from build123d import *

# Parameters (mm, degrees)
SKETCH1_R           = 12.5
BOSS_EXTRUDE1_DEPTH = 150
BOSS_EXTRUDE2_START = 5
SKETCH3_R           = 15.5
BOSS_EXTRUDE2_DEPTH = 10
CIRPATTERN1_COUNT   = 7
FILLET1_R           = 1


with BuildPart() as part:
    # Sketch1 → Boss-Extrude1 (new body)
    with BuildSketch(Plane(origin=(0, 0, 0), x_dir=(1, 0, 0), z_dir=(0, 1, 0))):
        Circle(SKETCH1_R)
    extrude(amount=BOSS_EXTRUDE1_DEPTH)

    # Sketch3 → Boss-Extrude2 (add)
    with BuildSketch(Plane(origin=(0, 0, 0), x_dir=(1, 0, 0), z_dir=(0, 1, 0)).offset(BOSS_EXTRUDE2_START)):
        with BuildLine():
            Line((-2.253835774, 56.947383215), (-2.253835774, 12.295130105))
            Line((-2.253835774, 12.295130105), (2.253835774, 12.295130105))
            Line((2.253835774, 12.295130105), (2.253835774, 56.947383215))
            ThreePointArc((2.253835774, 56.947383215), (0, 92.805720885), (-2.253835774, 56.947383215))
        make_face()
        with Locations((0, 74.805720885)):
            Circle(SKETCH3_R, mode=Mode.SUBTRACT)
    boss_extrude2 = extrude(amount=BOSS_EXTRUDE2_DEPTH)

    # CirPattern1: Boss-Extrude2 ×7 about axis
    cirpattern1_axis = Axis((0, 0, 0), (0, 1, 0))
    for i in range(1, CIRPATTERN1_COUNT):
        add(boss_extrude2.rotate(cirpattern1_axis, i * 360 / CIRPATTERN1_COUNT))

    # Fillet1
    fillet1_edges = [part.edges().sort_by_distance(p)[0] for p in [
        (-12.5, 0, 0),
    ]]
    fillet(fillet1_edges, radius=FILLET1_R)


solid = part.part
Can you work these out from the model? Positions are in its coordinate system, mm. A direction names the side the tool comes from. Give positions to 0.01 mm unless a question says otherwise; leave off trailing zeros. Order: outer loops, then holes, each group sorted by start corner. A loop starts at its lowest first (then second) coordinate and runs counter-clockwise, first axis right, second up. Notation, with made-up numbers: M 23,-19.5 L 58,-19.5 A26 ccw 58,8.5 Z; hole C 48,-17.5 d1. An arc over 180 degrees is marked long. Use a Markdown table: item, result. Add a question column.
Item 1: We'd pull the mould along Z, two halves only. Please class faces 1 (the flat face through (46, 5, -37)), 2 (the cylindrical face through (-87.526, 9.93, 11.43)): +Z half, -Z half, draft (parallel to the pull), parting line (faces both ways), or undercut.
Item 2: Suppose I cut it at C-C (y = 80). List the corners of the cut face in (x, z) for me, then the cut area to 3 significant figures.
Item 3: Suppose I cut it at A-A (z = -44.5). List the corners of the cut face in (x, y) for me, then the cut area to 3 significant figures.
Item 4: If I drill on L1, parallel to Z at x = -32, y = 7.5; L2, parallel to Y at x = 73, z = -1; L3, parallel to X at y = 69, z = -4, over which ranges is the centre line in solid material (lowest first)? Write a range as [from, to].
Item 5: Suppose I cut it at B-B (x = -38). List the corners of the cut face in (y, z) for me, then the cut area to 3 significant figures.
Item 6: Will these pins go through, and if not, where does the flat tip stop? pin 1 (1.5 mm diameter, centred on x = -11.5, z = -61.5, fed in from +Y); pin 2 (11 mm diameter, centred on y = 10.5, z = -26, fed in from -X); pin 3 (4 mm diameter, centred on x = 8.5, y = 122.5, fed in from -Z).
Item 7: For faces 3 (the flat face through (0, 0, 0)), 4 (the flat face through (0, 15, -59)), 5 (the flat face through (-33.56, 9.93, 9.97)), which set-ups out of +Z, -Z, +X, -X, +Y, -Y let a thin tool reach every point of the face, with its end or its side?
Answer sheet:
| question | item | result |
|---|---|---|
| 1 | face 1 | draft |
| 1 | face 2 | undercut |
| 2 | outline | C 0,0 d25 |
| 2 | area | 491 mm² |
| 3 | outline | M -76.36,5 L -73.84,5 L -73.84,15 L -76.36,15 Z; M -43.13,5 L -40.61,5 L -40.61,15 L -43.13,15 Z; M -2.25,5 L 2.25,5 L 2.25,15 L -2.25,15 Z; M 40.61,5 L 43.13,5 L 43.13,15 L 40.61,15 Z; M 73.84,5 L 76.36,5 L 76.36,15 L 73.84,15 Z |
| 3 | area | 146 mm² |
| 4 | L1 | z = [-28.4, -22.64], [4.99, 9.62], [49.4, 51.9], [82.89, 85.39] |
| 4 | L2 | y = [5, 15] |
| 4 | L3 | x = [-11.84, 11.84] |
| 5 | outline | M 5,-33.19 L 15,-33.19 L 15,-27.42 L 5,-27.42 Z; M 5,6.36 L 15,6.36 L 15,10.99 L 5,10.99 Z; M 5,50.27 L 15,50.27 L 15,52.92 L 5,52.92 Z; M 5,81.87 L 15,81.87 L 15,84.52 L 5,84.52 Z |
| 5 | area | 157 mm² |
| 6 | pin 1 | stops at y = 15 |
| 6 | pin 2 | stops at x = -68.22 |
| 6 | pin 3 | stops at z = -10.68 |
| 7 | face 3 | +Z, -Z, +X, -X, -Y |
| 7 | face 4 | -Z, +X, -X, +Y |
| 7 | face 5 | +Y, -Y |
